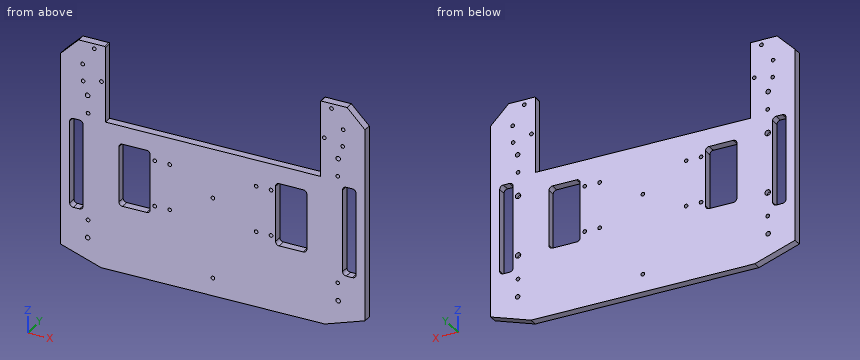
```python
from build123d import *

# Parameters (mm, degrees)
ESQUISSE3_R          = 2.55
STRUCTURE_DEPTH      = 9
ESQUISSE4_R          = 3.05
ENCOCHES_TIGES_DEPTH = 5
ESQUISSE5_R          = 2.05
ENCODEURS_DEPTH      = 221.410979763
MOTEURS_DEPTH        = 221.410979763
MOTEURS_DEPTH_BACK   = 221.410979763
ESQUISSE6_R          = 2.05
ESQUISSE7_R          = 2.05
PATINS_DEPTH         = 221.410979763
ESQUISSE8_R          = 2.05
ACTIONNEURS_DEPTH    = 221.410979763
CONG_1_R             = 1


with BuildPart() as part:
    # Esquisse3 → structure (new body)
    with BuildSketch(Plane(origin=(0, 0, 0), x_dir=(1, 0, 0), z_dir=(0, 1, 0))):
        Polygon((125, 110), (-125, 110), (-170, 95), (-170, 0), (-170, -120), (-150, -140), (-120, -140), (-120, -55), (120, -55), (120, -140), (150, -140), (170, -120), (170, 0), (170, 95), align=None)
        with Locations(Location((-140, 80, 0), (0, 0, 270))):
            Circle(ESQUISSE3_R, mode=Mode.SUBTRACT)
        with Locations(Location((-140, -80, 0), (0, 0, 90))):
            Circle(ESQUISSE3_R, mode=Mode.SUBTRACT)
        with Locations(Location((140, -80, 0), (0, 0, 270))):
            Circle(ESQUISSE3_R, mode=Mode.SUBTRACT)
        with Locations(Location((140, 80, 0), (0, 0, 90))):
            Circle(ESQUISSE3_R, mode=Mode.SUBTRACT)
        with BuildLine():
            Line((-160, -46), (-160, 46))
            ThreePointArc((-160, 46), (-158.828427125, 48.828427125), (-156, 50))
            Line((-156, 50), (-149, 50))
            ThreePointArc((-149, 50), (-146.171572875, 48.828427125), (-145, 46))
            Line((-145, 46), (-145, -46))
            ThreePointArc((-145, -46), (-146.171572875, -48.828427125), (-149, -50))
            Line((-149, -50), (-156, -50))
            ThreePointArc((-156, -50), (-158.828427125, -48.828427125), (-160, -46))
        make_face(mode=Mode.SUBTRACT)
        with BuildLine():
            Line((-105, 0), (-105, 31))
            ThreePointArc((-105, 31), (-103.828427125, 33.828427125), (-101, 35))
            Line((-101, 35), (-74, 35))
            ThreePointArc((-74, 35), (-71.171572875, 33.828427125), (-70, 31))
            Line((-70, 31), (-70, -31))
            ThreePointArc((-70, -31), (-71.171572875, -33.828427125), (-74, -35))
            Line((-74, -35), (-101, -35))
            ThreePointArc((-101, -35), (-103.828427125, -33.828427125), (-105, -31))
            Line((-105, -31), (-105, 0))
        make_face(mode=Mode.SUBTRACT)
        with BuildLine():
            Line((156, 50), (149, 50))
            ThreePointArc((149, 50), (146.171572875, 48.828427125), (145, 46))
            Line((145, 46), (145, -46))
            ThreePointArc((145, -46), (146.171572875, -48.828427125), (149, -50))
            Line((149, -50), (156, -50))
            ThreePointArc((156, -50), (158.828427125, -48.828427125), (160, -46))
            Line((160, -46), (160, 46))
            ThreePointArc((160, 46), (158.828427125, 48.828427125), (156, 50))
        make_face(mode=Mode.SUBTRACT)
        with BuildLine():
            Line((105, 0), (105, 31))
            ThreePointArc((105, 31), (103.828427125, 33.828427125), (101, 35))
            Line((101, 35), (74, 35))
            ThreePointArc((74, 35), (71.171572875, 33.828427125), (70, 31))
            Line((70, 31), (70, -31))
            ThreePointArc((70, -31), (71.171572875, -33.828427125), (74, -35))
            Line((74, -35), (101, -35))
            ThreePointArc((101, -35), (103.828427125, -33.828427125), (105, -31))
            Line((105, -31), (105, 0))
        make_face(mode=Mode.SUBTRACT)
    extrude(amount=-STRUCTURE_DEPTH)

    # Esquisse4 → encoches_tiges (cut)
    with BuildSketch(Plane(origin=(0, 0, 0), x_dir=(1, 0, 0), z_dir=(0, 1, 0))):
        with Locations(Location((-139.5, 33.5, 0), (0, 0, 270))):
            Circle(ESQUISSE4_R)
        with Locations(Location((-139.5, -33.5, 0), (0, 0, 90))):
            Circle(ESQUISSE4_R)
        with Locations(Location((139.5, -33.5, 0), (0, 0, 270))):
            Circle(ESQUISSE4_R)
        with Locations(Location((139.5, 33.5, 0), (0, 0, 90))):
            Circle(ESQUISSE4_R)
    extrude(amount=-ENCOCHES_TIGES_DEPTH, mode=Mode.SUBTRACT)

    # Esquisse5 → encodeurs (cut, through all)
    with BuildSketch(Plane(origin=(0, 0, 0), x_dir=(1, 0, 0), z_dir=(0, 1, 0))):
        with Locations(Location((-139.5, 60, 0), (0, 0, 270))):
            Circle(ESQUISSE5_R)
        with Locations(Location((-139.5, -60, 0), (0, 0, 90))):
            Circle(ESQUISSE5_R)
        with Locations(Location((139.5, -60, 0), (0, 0, 270))):
            Circle(ESQUISSE5_R)
        with Locations(Location((139.5, 60, 0), (0, 0, 90))):
            Circle(ESQUISSE5_R)
    extrude(amount=-ENCODEURS_DEPTH, mode=Mode.SUBTRACT)

    # Esquisse6 → moteurs (cut, two sides: drawn at the far end of the back side and taken through both)
    with BuildSketch(Plane(origin=(0, 0, 0), x_dir=(1, 0, 0), z_dir=(0, 1, 0)).offset(-MOTEURS_DEPTH_BACK)):
        with Locations(Location((-65, 25.5, 0), (0, 0, 270))):
            Circle(ESQUISSE6_R)
        with Locations(Location((-48.3, 25.5, 0), (0, 0, 270))):
            Circle(ESQUISSE6_R)
        with Locations(Location((-65, -25.5, 0), (0, 0, 270))):
            Circle(ESQUISSE6_R)
        with Locations(Location((48.3, -25.5, 0), (0, 0, 270))):
            Circle(ESQUISSE6_R)
        with Locations(Location((65, -25.5, 0), (0, 0, 270))):
            Circle(ESQUISSE6_R)
        with Locations(Location((-48.3, -25.5, 0), (0, 0, 90))):
            Circle(ESQUISSE6_R)
        with Locations(Location((48.3, 25.5, 0), (0, 0, 90))):
            Circle(ESQUISSE6_R)
        with Locations(Location((65, 25.5, 0), (0, 0, 90))):
            Circle(ESQUISSE6_R)
    extrude(amount=MOTEURS_DEPTH + MOTEURS_DEPTH_BACK, mode=Mode.SUBTRACT)

    # Esquisse7 → patins (cut, through all)
    with BuildSketch(Plane(origin=(0, 0, 0), x_dir=(1, 0, 0), z_dir=(0, 1, 0))):
        with Locations(Location((0, 90, 0), (0, 0, 270))):
            Circle(ESQUISSE7_R)
        with Locations(Location((0, 0, 0), (0, 0, 270))):
            Circle(ESQUISSE7_R)
        with Locations(Location((-145, -95, 0), (0, 0, 270))):
            Circle(ESQUISSE7_R)
        with Locations(Location((145, -95, 0), (0, 0, 90))):
            Circle(ESQUISSE7_R)
    extrude(amount=-PATINS_DEPTH, mode=Mode.SUBTRACT)

    # Esquisse8 → actionneurs (cut, through all)
    with BuildSketch(Plane(origin=(0, 0, 0), x_dir=(1, 0, 0), z_dir=(0, 1, 0))):
        with Locations(Location((-132.5, -134.5, 0), (0, 0, 270))):
            Circle(ESQUISSE8_R)
        with Locations(Location((-124.5, -99.5, 0), (0, 0, 270))):
            Circle(ESQUISSE8_R)
        with Locations(Location((132.5, -134.5, 0), (0, 0, 90))):
            Circle(ESQUISSE8_R)
        with Locations(Location((124.5, -99.5, 0), (0, 0, 90))):
            Circle(ESQUISSE8_R)
        with Locations(Location((-145.5, -114, 0), (0, 0, 270))):
            Circle(ESQUISSE8_R)
        with Locations(Location((145.5, -114, 0), (0, 0, 90))):
            Circle(ESQUISSE8_R)
    extrude(amount=-ACTIONNEURS_DEPTH, mode=Mode.SUBTRACT)

    # Congé1
    cong_1_edges = [part.edges().sort_by_distance(p)[0] for p in [
        (-120, -4.5, 140),
        (120, -4.5, 140),
    ]]
    fillet(cong_1_edges, radius=CONG_1_R)


solid = part.part
```
Work out the finished part from the listing and answer in its coordinate system (mm). Give positions to 0.01 mm unless a question says otherwise; leave off trailing zeros. Write each loop counter-clockwise with the first axis right and the second up, starting at its lowest first coordinate (ties: lowest second). Pieces come first, ordered by that corner, then holes. Notation, with made-up numbers: (49.5, 76) -> (66.5, 76) arc R31 cw to (66.5, 104) -> close; hole circle Ø11 at (-13, -10). An arc over 180 degrees is marked (long way). Write item = value, one per line.
Q1. Flat-ended cylindrical pins translate along their axes: pin 1 Ø3 at (x, z) = (-140, -80) entering from +Y; pin 2 Ø2 at (x, y) = (-22.5, -7.5) entering from +Z. Find the tip coordinate at first contact, or state that the pin passes through.
Computed values:
pin_1 = through
pin_2 = 55
Q2. Section A-A on y = -2.5 is taken. State how many separate pieces and enclosed holes the cut face has, and give its area (3 significant figures).
Computed values:
separate_pieces = 1
enclosed_holes = 34
area = 55,200 mm^2
Q3. Section B-B on x = -34 is taken. Determine the outline of the cut face in (y, z), and give its area (4 significant figures).
Computed values:
outline = (-9, -110) -> (0, -110) -> (0, 55) -> (-9, 55) -> close
area = 1,485 mm^2
Q4. Consider line 1 along X through (y, z) = (-7.25, 45.5); line 2 along X through (y, z) = (-5.75, -30.5); line 3 along X through (y, z) = (-5.5, -80). Determine where each line is inside the solid, lowest interval first.
Computed values:
line_1 = -170 to -160, -145 to 145, 160 to 170
line_2 = -170 to -160, -145 to -105, -70 to 70, 105 to 145, 160 to 170
line_3 = -170 to -142.55, -137.45 to 137.45, 142.55 to 170
